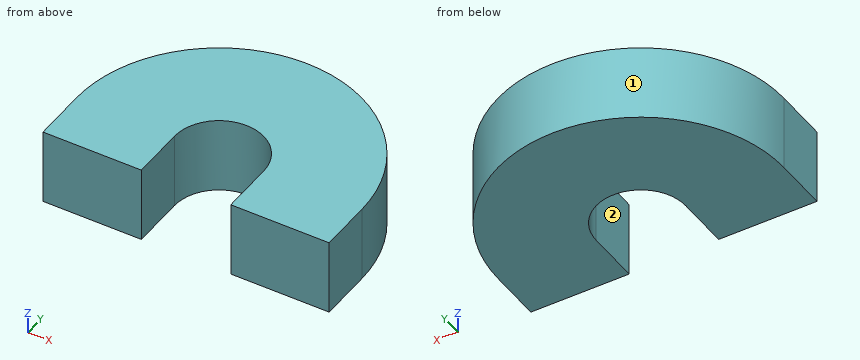
Autodesk Inventor part; units mm, degrees
ref_plane "YZ Plane" through (0, 0, 0) normal (1, 0, 0) x (0, 1, 0)
ref_plane "XZ Plane" through (0, 0, 0) normal (0, 1, 0) x (-1, 0, 0)
ref_plane "XY Plane" through (0, 0, 0) normal (0, 0, 1) x (1, 0, 0)
sketch "Sketch1" plane through (0, 0, 0) normal (0, 0, 1) x (1, 0, 0)
  circle A0 centre (0, 0) radius 2.5
  circle A1 centre (0, 0) radius 8
  line L0 (-8, 0) -> (8, 0)
  point P0 (-2.5, 0)
  point P1 (2.5, 0)
  dimension "d0" = 16
  dimension "d1" = 5
extrude "Extrusion1" add sketch "Sketch1" along normal blind 4.25 contours A0 L0 A1 picked at (-6.065, 0.8376)
sketch "Sketch2" plane through (-8, 0, 0) normal (0, -1, 0) x (1, 0, 0)
  line L0 (0, 0) -> (5.5, 0)
  line L1 (5.5, 0) -> (5.5, 4.25)
  line L2 (0, 4.25) -> (5.5, 4.25)
  line L3 (0, 0) -> (0, 4.25)
  line L4 (10.5, 0) -> (16, 0)
  line L5 (16, 0) -> (16, 4.25)
  line L6 (10.5, 4.25) -> (16, 4.25)
  line L7 (10.5, 0) -> (10.5, 4.25)
  point P0 (8, 0)
extrude "Extrusion2" add sketch "Sketch2" along normal blind 3
properties part number "Riemenscheibe_Adjustment_Disk"
The listing builds one solid part. Answer for the finished solid, in the listing's coordinates (mm). Face numbers are marked on the shaded views. A direction names the side the tool comes from. Round coordinates to 2 decimals unless told otherwise and drop trailing zeros. Write each loop counter-clockwise with the first axis right and the second up, starting at its lowest first coordinate (ties: lowest second). Pieces come first, ordered by that corner, then holes. Notation, with made-up numbers: M 47.5,62 L 106.5,62 A15 cw 106.5,79 Z; hole C 29.5,38 d10. An arc over 180 degrees is marked long. Write each question's results on one line, items separated by ' | '. Start each with the question number.
Item 1: Straight lines are drawn through the part: probe 1 along X at (y, z) = (-0.75, 0.8); probe 2 along X at (y, z) = (2, 1.95); probe 3 along Y at (x, z) = (0, 3.15). For each, find the intervals that lie inside material, in ascending order.
Item 2: Which of the six approach directions +Z, -Z, +X, -X, +Y, -Y give full straight-line access (tool end or side, diameter ignored) to the marked faces 1 and 2?
Item 3: Given pin 1 Ø2 at (x, z) = (5.5, 3) entering from +Y, flat-ended and moving along its own axis, determine where the tip first touches the part or whether it passes through.
Item 4: Find section B-B on x = 0. Write down the section's boundary in (y, z).
Item 5: Find section A-A on z = 0.55. Write down the section's boundary in (x, y).
Item 6: Find section C-C on y = 4.5. Write down the section's boundary in (x, z).
Answer block:
1) probe 1: x = -8 to -2.5, 2.5 to 8 | probe 2: x = -7.75 to -1.5, 1.5 to 7.75 | probe 3: y = 2.5 to 8
2) face 1: +Z, -Z, +Y | face 2: +Z, -Z, -Y
3) pin 1: stops at y = 6.61
4) outline: M 2.5,0 L 8,0 L 8,4.25 L 2.5,4.25 Z
5) outline: M -8,-3 L -2.5,-3 L -2.5,0 A2.5 cw 2.5,0 L 2.5,-3 L 8,-3 L 8,0 A8 ccw -8,0 Z
6) outline: M -6.61,0 L 6.61,0 L 6.61,4.25 L -6.61,4.25 Z
